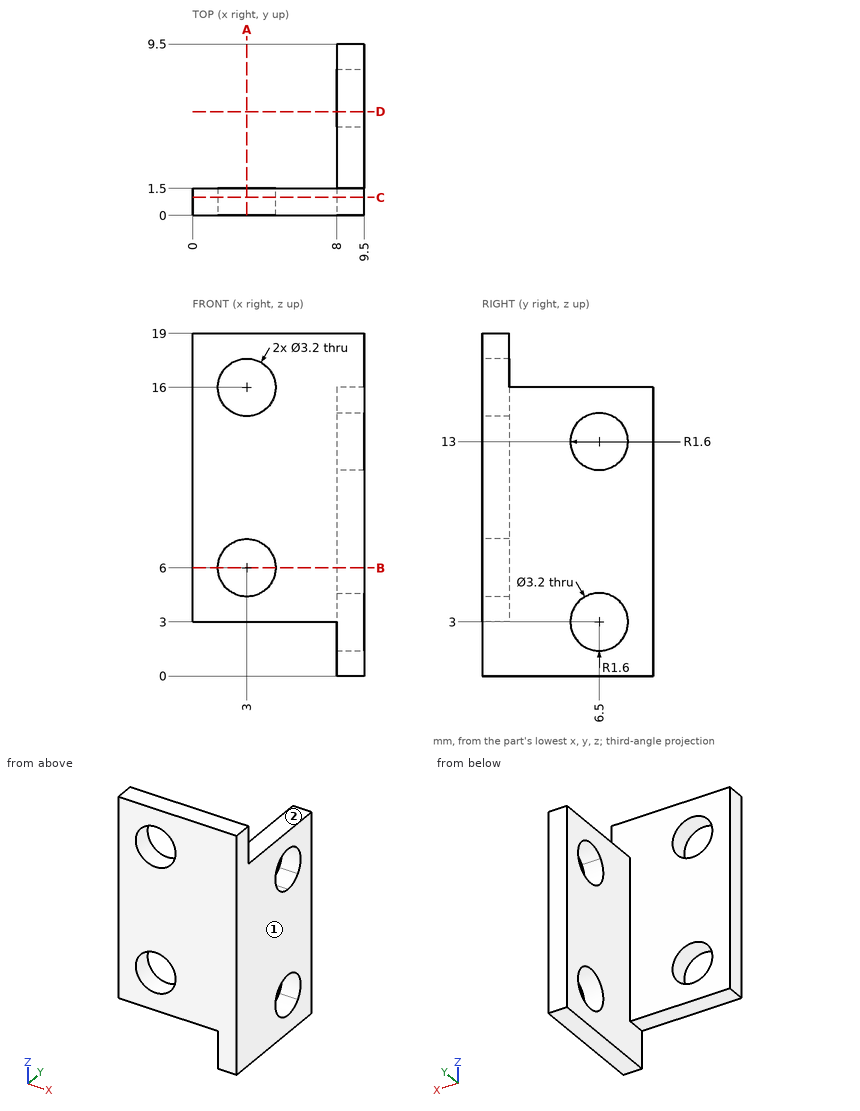
For this review, use the dimensioned drawing (mm, ordinates from the lowest corner) and the shaded views. A direction names the side the tool comes from. Round coordinates to 2 decimals unless told otherwise and drop trailing zeros. Loops run counter-clockwise (first coordinate to the right, second up) from the corner with the lowest first, then second, coordinate; pieces in that order, holes last. Notation, with made-up numbers: M 88.5,6.25 L 141.5,6.25 A29 ccw 141.5,36.25 Z; hole C 71.5,67 d11. An arc over 180 degrees is marked long. Answer as CSV lines item,"result".
1. We need section D-D (y = 5.75). Give the boundary of the cut face in (x, z).
Outcome:
outline,"M 8,0 L 9.5,0 L 9.5,1.59 L 8,1.59 Z; M 8,4.41 L 9.5,4.41 L 9.5,11.59 L 8,11.59 Z; M 8,14.41 L 9.5,14.41 L 9.5,16 L 8,16 Z"
2. To check wall thickness, follow L1, parallel to Z at x = 3, y = 0.65; L2, parallel to Y at x = 8.5, z = 3; L3, parallel to X at y = 3.25, z = 6.25. State the ranges of each line that lie inside material, in increasing order. Write a range as [from, to].
Outcome:
L1,"z = [3, 4.4], [7.6, 14.4], [17.6, 19]"
L2,"y = [0, 4.9], [8.1, 9.5]"
L3,"x = [8, 9.5]"
3. We need section C-C (y = 1). Give the boundary of the cut face in (x, z).
Outcome:
outline,"M 0,3 L 8,3 L 8,0 L 9.5,0 L 9.5,19 L 0,19 Z; hole C 3,6 d3.2; hole C 3,16 d3.2"
4. We need section B-B (z = 6). Give the boundary of the cut face in (x, y).
Outcome:
outline,"M 0,0 L 1.4,0 L 1.4,1.5 L 0,1.5 Z; M 4.6,0 L 9.5,0 L 9.5,9.5 L 8,9.5 L 8,1.5 L 4.6,1.5 Z"
5. For the marked faces 1 and 2, list the 3-axis set-ups (+Z, -Z, +X, -X, +Y, -Y) from which the entire face can be reached by the end or side of a thin tool; tool diameter is ignored.
Outcome:
face 1,"+Z, -Z, +X, +Y, -Y"
face 2,"+Z, +X, -X, +Y"
6. We need section A-A (x = 3). Give the boundary of the cut face in (y, z), plus the area to 3 significant figures.
Outcome:
outline,"M 0,3 L 1.5,3 L 1.5,4.4 L 0,4.4 Z; M 0,7.6 L 1.5,7.6 L 1.5,14.4 L 0,14.4 Z; M 0,17.6 L 1.5,17.6 L 1.5,19 L 0,19 Z"
area,"14.4 mm2"
7. Insertion check: pin 1 Ø0.8 at (x, y) = (8.5, 4.5) entering from +Z; pin 2 Ø3.5 at (x, z) = (3, 6) entering from +Y; pin 3 Ø1.2 at (x, y) = (3.5, 1) entering from -Z. Each pin has a flat end and moves straight along its axis. Give the tip position at first contact, or say it passes through.
Outcome:
pin 1,"stops at z = 16"
pin 2,"stops at y = 1.5"
pin 3,"stops at z = 3"
